Model file for the job. Use its own axes, mm. A direction names the side the tool comes from. Round coordinates to 2 decimals unless told otherwise and drop trailing zeros. Loops run counter-clockwise (first coordinate to the right, second up) from the corner with the lowest first, then second, coordinate; pieces in that order, holes last.
from build123d import *

# Parameters (mm, degrees)
SKETCH1_W               = 400
SKETCH1_H               = 600
BOSS_EXTRUDE1_DEPTH     = 9.525
F_1_4_CLEARANCE_HOLE1_D = 7.14248
LPATTERN1_COUNT         = 2
LPATTERN1_PITCH         = 50.8
CUT_EXTRUDE2_DEPTH      = 10.525
LPATTERN2_COUNT         = 3
LPATTERN2_PITCH         = 76.2
LPATTERN2_COL_COUNT     = 3
LPATTERN2_COL_PITCH     = 76.2
SKETCH6_W               = 300
SKETCH6_H               = 250
SKETCH6_H_2             = 100
CUT_EXTRUDE1_DEPTH      = 10.525
SKETCH7_W               = 50
SKETCH7_H               = 410
BOSS_EXTRUDE2_DEPTH     = 9.525
FILLET1_R               = 25
CHAMFER2_SIZE           = 3


with BuildPart() as part:
    # Sketch1 → Boss-Extrude1 (new body)
    with BuildSketch(Plane.XY):
        with Locations((0, 300)):
            Rectangle(SKETCH1_W, SKETCH1_H)
    extrude(amount=BOSS_EXTRUDE1_DEPTH)

    # 1/4 Clearance Hole1 (through all)
    with Locations(Plane.XY.offset(9.525)):
        with Locations((-175, 12.7), (-175, 38.1), (175, 38.1), (175, 12.7), (0, 38.1), (0, 12.7)):
            f_1_4_clearance_hole1 = Hole(F_1_4_CLEARANCE_HOLE1_D / 2)

    # LPattern1: 1/4 Clearance Hole1 ×2
    with Locations(*[(0, i * LPATTERN1_PITCH, 0) for i in range(1, LPATTERN1_COUNT)]):
        add(f_1_4_clearance_hole1, mode=Mode.SUBTRACT)

    # Sketch8 → Cut-Extrude2 (cut, through all)
    with BuildSketch(Plane.XY.offset(9.525)):
        with BuildLine():
            Line((-17.5, 582.5), (17.5, 582.5))
            ThreePointArc((17.5, 582.5), (25, 575), (17.5, 567.5))
            Line((17.5, 567.5), (-17.5, 567.5))
            ThreePointArc((-17.5, 567.5), (-25, 575), (-17.5, 582.5))
        make_face()
    cut_extrude2 = extrude(amount=-CUT_EXTRUDE2_DEPTH, mode=Mode.SUBTRACT)

    # LPattern2: Cut-Extrude2 ×3
    with Locations(*[(i * LPATTERN2_PITCH, 0, 0) for i in range(1, LPATTERN2_COUNT)]):
        add(cut_extrude2, mode=Mode.SUBTRACT)

    # LPattern2 col: Cut-Extrude2 ×3
    with Locations(*[(-i * LPATTERN2_COL_PITCH, 0, 0) for i in range(1, LPATTERN2_COL_COUNT)]):
        add(cut_extrude2, mode=Mode.SUBTRACT)

    # Sketch6 → Cut-Extrude1 (cut, through all)
    with BuildSketch(Plane.XY.offset(9.525)):
        with Locations((0, 255)):
            Rectangle(SKETCH6_W, SKETCH6_H)
        with Locations((0, 490)):
            Rectangle(SKETCH6_W, SKETCH6_H_2)
    extrude(amount=-CUT_EXTRUDE1_DEPTH, mode=Mode.SUBTRACT)

    # Sketch7 → Boss-Extrude2 (add, through all)
    with BuildSketch(Plane.XY.offset(9.525)):
        with Locations((0, 335)):
            Rectangle(SKETCH7_W, SKETCH7_H)
    extrude(amount=-BOSS_EXTRUDE2_DEPTH)

    # Fillet1
    fillet1_edges = [part.edges().sort_by_distance(p)[0] for p in [
        (-150, 130, 4.7625),
        (-150, 380, 4.7625),
        (150, 380, 4.7625),
        (150, 130, 4.7625),
        (-150, 440, 4.7625),
        (-150, 540, 4.7625),
        (150, 540, 4.7625),
        (150, 440, 4.7625),
        (-25, 440, 4.7625),
        (25, 440, 4.7625),
        (25, 540, 4.7625),
        (-25, 130, 4.7625),
        (-25, 540, 4.7625),
        (25, 380, 4.7625),
        (25, 130, 4.7625),
        (-25, 380, 4.7625),
    ]]
    fillet(fillet1_edges, radius=FILLET1_R)

    # Chamfer2
    chamfer2_edges = [part.edges().sort_by_distance(p)[0] for p in [
        (-200, 600, 4.7625),
        (200, 600, 4.7625),
        (200, 0, 4.7625),
        (-200, 0, 4.7625),
    ]]
    chamfer(chamfer2_edges, length=CHAMFER2_SIZE)


solid = part.part
Q1. Slice it at D-D on z = 3.25. State how many separate pieces and enclosed holes the cut face has, plus the area to 3 significant figures.
Q2. Slice it at B-B on x = 156.5. Give the cut face in (y, z) (3 decimals).
Q3. Flat gauge pin, fed straight in: P1, Ø6.5, axis at x = 175, y = 12.7, coming from the -Z side (3 decimals). Where does the tip first touch, or does it go through?
Q4. Pull direction Y, two halves, no side cores. Call faces 1 (the face through (-142.482, 532.871, 4.696)), 2 (the face through (-32.518, 532.871, 4.696)), 3 (the face through (-3, 238, 9.525)): pulls with the +Y half, pulls with the -Y half, needs draft (parallel to the pull), parting line crosses it, or undercut.
Q5. Tool access for faces 4 (the face through (-3, 238, 0)), 5 (the face through (142.871, 532.482, 4.696)): list every direction of +Z, -Z, +X, -X, +Y, -Y with a clear straight run to the whole face (end or side of a thin tool).
Q6. Slice it at A-A on x = 64.5. Give the cut face in (y, z) (3 decimals).
Q7. Probe line 1 (Y direction, x = -71, z = 5); line 2 (X direction, y = 63, z = 6.25); line 3 (X direction, y = 463, z = 7.75). List the from-to ranges inside material, lowest first.
Q8. Slice it at C-C on y = 362.5. Give the cut face in (x, z) (3 decimals), plus the area to 3 significant figures.
Reply:
1. separate pieces: 1
1. enclosed holes: 21
1. area: 151,000 mm2
2. outline: (0, 0) - (567.5, 0) - (567.5, 9.525) - (0, 9.525) - close; (582.5, 0) - (600, 0) - (600, 9.525) - (582.5, 9.525) - close
3. P1: passes through
4. face 1: undercut
4. face 2: undercut
4. face 3: needs draft
5. face 4: -Z, +X, -X, +Y, -Y
5. face 5: +Z, -Z
6. outline: (0, 0) - (130, 0) - (130, 9.525) - (0, 9.525) - close; (380, 0) - (440, 0) - (440, 9.525) - (380, 9.525) - close; (540, 0) - (567.5, 0) - (567.5, 9.525) - (540, 9.525) - close; (582.5, 0) - (600, 0) - (600, 9.525) - (582.5, 9.525) - close
7. line 1: y = 0 to 130, 380 to 440, 540 to 567.5, 582.5 to 600
7. line 2: x = -200 to -178.54, -171.46 to -3.54, 3.54 to 171.46, 178.54 to 200
7. line 3: x = -200 to -149.92, -25.08 to 25.08, 149.92 to 200
8. outline: (-200, 0) - (-148.848, 0) - (-148.848, 9.525) - (-200, 9.525) - close; (-26.152, 0) - (26.152, 0) - (26.152, 9.525) - (-26.152, 9.525) - close; (148.848, 0) - (200, 0) - (200, 9.525) - (148.848, 9.525) - close
8. area: 1,470 mm2
